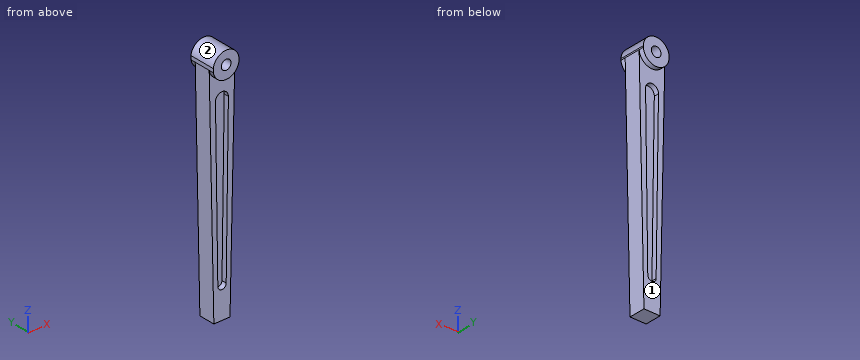
from build123d import *

# Parameters (mm, degrees)
F1_DEPTH = 2.5
F0_R     = 1.5
F2_DEPTH = 4
F3_DEPTH = 1


# Not quite as in the source:
# - a feature names something its author has since deleted; it is built from what else it names


with BuildPart() as f1:
    # F0 (on Front) → F1 (new body, symmetric)
    with BuildSketch(Plane.XZ):
        with BuildLine():
            Line((-3.9449856715, 23.9478669513), (-2.5, -45.3910091387))
            Line((-2.5, -45.3910091387), (2.5, -45.3910091387))
            Line((2.5, -45.3910091387), (3.9887932138, 24.3097798378))
            ThreePointArc((3.9887932138, 24.3097798378), (0.1822772875, 20.6131485868), (-3.9449856715, 23.9478669513))
        make_face()
        with BuildLine():
            ThreePointArc((-1.9997903124, 14.6349845216), (-0.0009328581, 16.6639447346), (1.9998164582, 14.6368500546))
            Line((1.9998164582, 14.6368500546), (1.3173793796, -35.7323714856))
            ThreePointArc((1.3173793796, -35.7323714856), (0.0241016903, -37.0088409461), (-1.270366201, -35.7335784854))
            Line((-1.270366201, -35.7335784854), (-1.9997903124, 14.6349845216))
        make_face(mode=Mode.SUBTRACT)
    extrude(amount=F1_DEPTH, both=True)

    # F0 (on Front) → F2 (join, symmetric)
    with BuildSketch(Plane.XZ):
        with BuildLine():
            Line((-3.9691037619, 25.1051941963), (-3.9449856715, 23.9478669513))
            ThreePointArc((-3.9449856715, 23.9478669513), (0.1822772875, 20.6131485868), (3.9887932138, 24.3097798378))
            Line((3.9887932138, 24.3097798378), (3.9979316153, 24.7376121165))
            ThreePointArc((3.9979316153, 24.7376121165), (0.184355384, 28.6047426804), (-3.9691037619, 25.1051941963))
        make_face()
        with Locations((0, 24.6089933023)):
            Circle(F0_R, mode=Mode.SUBTRACT)
    extrude(amount=F2_DEPTH, both=True)

    # F0 (on Front) → F3 (join, symmetric)
    with BuildSketch(Plane.XZ):
        with BuildLine():
            Line((1.3173793796, -35.7323714856), (1.9998164582, 14.6368500546))
            ThreePointArc((1.9998164582, 14.6368500546), (-0.0009328581, 16.6639447346), (-1.9997903124, 14.6349845216))
            Line((-1.9997903124, 14.6349845216), (-1.270366201, -35.7335784854))
            ThreePointArc((-1.270366201, -35.7335784854), (0.0241016903, -37.0088409461), (1.3173793796, -35.7323714856))
        make_face()
    extrude(amount=F3_DEPTH, both=True)


solid = f1.part
CAD build for the part. Positions are in the model's coordinates, mm. Face numbers are marked on the shaded views. Round coordinates to 2 decimals unless told otherwise and drop trailing zeros. Order: outer loops, then holes, each group sorted by start corner. A loop starts at its lowest first (then second) coordinate and runs counter-clockwise, first axis right, second up. Notation, with made-up numbers: (68.5, 61.25) -> (93.5, 61.25) arc R26 ccw to (93.5, 99.25) -> close; hole circle Ø11 at (75.25, 55.5). An arc over 180 degrees is marked (long way). Write item = value, one per line. Start each with the question number.
(1) Probe line 1 (Z direction, x = 0, y = -1.25); line 2 (Y direction, x = 3.5, z = 15); line 3 (Y direction, x = 0, z = -5). List the from-to ranges inside material, lowest first. Write a range as [from, to].
(2) Cut at C-C, the plane y = 0. List the corners of the cut face in (x, z).
(3) Cut at D-D, the plane z = -3. List the corners of the cut face in (x, y), then the cut area to 3 significant figures.
(4) Pull direction Z, two halves, no side cores. Call the marked faces 1 and 2: released by +Z, released by -Z, zero draft, split by the parting line, or undercut.
(5) Cut at A-A, the plane x = 0. List the corners of the cut face in (y, z), then the cut area to 3 significant figures.
(6) Pin check, flat tips, straight feed: P1, Ø2.5, axis at x = 0, z = 24.61, coming from the -Y side; P2, Ø4.5, axis at x = -0.5, z = -11, coming from the +Y side; P3, Ø3, axis at x = 1.5, z = -5, coming from the -Y side; P4, Ø1.2, axis at x = 0.5, z = 0, coming from the -Y side. Stop position of each tip, or through.
(7) Cut at B-B, the plane z = -27.5. List the corners of the cut face in (x, y), then the cut area to 3 significant figures.
Model answer:
q1.line_1 = [-45.39, -37.01], [16.66, 23.11], [26.11, 28.61]
q1.line_2 = [-2.5, 2.5]
q1.line_3 = [-1, 1]
q2.outline = (-3.97, 25.11) -> (-2.5, -45.39) -> (2.5, -45.39) -> (4, 24.74) arc R4 ccw to start; hole circle Ø3 at (0, 24.61)
q3.outline = (-3.38, -2.5) -> (-1.74, -2.5) -> (-1.74, -1) -> (1.76, -1) -> (1.76, -2.5) -> (3.41, -2.5) -> (3.41, 2.5) -> (1.76, 2.5) -> (1.76, 1) -> (-1.74, 1) -> (-1.74, 2.5) -> (-3.38, 2.5) -> close
q3.area = 23.4 mm2
q4.face_1 = zero draft
q4.face_2 = released by +Z
q5.outline = (-4, 20.61) -> (-2.5, 20.61) -> (-2.5, 16.66) -> (-1, 16.66) -> (-1, -37.01) -> (-2.5, -37.01) -> (-2.5, -45.39) -> (2.5, -45.39) -> (2.5, -37.01) -> (1, -37.01) -> (1, 16.66) -> (2.5, 16.66) -> (2.5, 20.61) -> (4, 20.61) -> (4, 23.11) -> (-4, 23.11) -> close; (-4, 26.11) -> (4, 26.11) -> (4, 28.61) -> (-4, 28.61) -> close
q5.area = 209 mm2
q6.P1 = through
q6.P2 = 2.5
q6.P3 = -2.5
q6.P4 = -1
q7.outline = (-2.87, -2.5) -> (-1.39, -2.5) -> (-1.39, -1) -> (1.43, -1) -> (1.43, -2.5) -> (2.88, -2.5) -> (2.88, 2.5) -> (1.43, 2.5) -> (1.43, 1) -> (-1.39, 1) -> (-1.39, 2.5) -> (-2.87, 2.5) -> close
q7.area = 20.3 mm2
